Geometry: see drawing. Coordinates: mm, zero at the bounding-box minimum. Coordinates: 2 decimals unless noted, no trailing zeros. Write each loop counter-clockwise with the first axis right and the second up, starting at its lowest first coordinate (ties: lowest second). Pieces come first, ordered by that corner, then holes. Notation, with made-up numbers: (89.25, 1.25) - (126.25, 1.25) arc R14 ccw to (126.25, 27.25) - close; hole circle Ø6 at (21.25, 2). An arc over 180 degrees is marked (long way). Use CSV: the item, a comma, the result in double quotes.
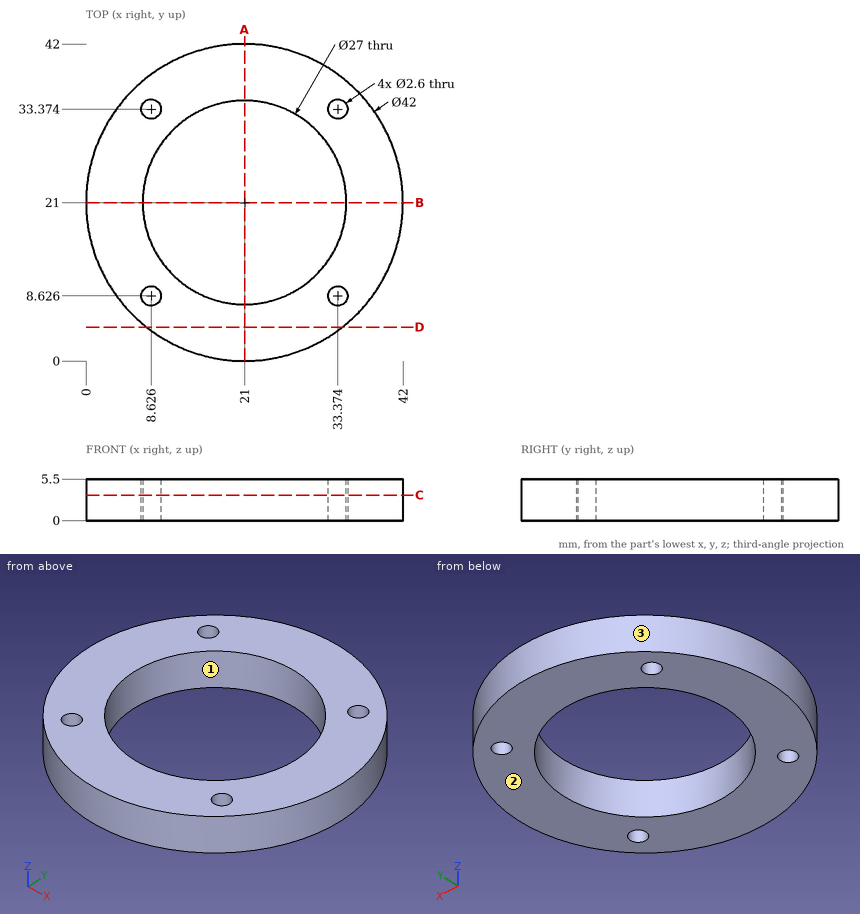
(1) Draft query along Y for the marked faces 1, 2 and 3. Return one class per face: pulls with the +Y half, pulls with the -Y half, needs draft (parallel to the pull), parting line crosses it, or undercut.
Check values:
face 1,"undercut"
face 2,"needs draft"
face 3,"parting line crosses it"
(2) Pin query (flat end, axial travel): pin 1 Ø3 at (x, z) = (32, 2) entering from +Y; pin 2 Ø2 at (x, z) = (24, 1) entering from -Y (1 decimal); pin 3 Ø2 at (x, z) = (9.5, 4.5) entering from +Y. Return the tip coordinate at first contact, or that it passes through.
Check values:
pin 1,"y = 39.73"
pin 2,"y = 0.1"
pin 3,"y = 39.19"
(3) Cut plane C-C on z = 3.35. Return loops of the section in (x, y) (1 decimal).
Check values:
outline,"circle Ø42 at (21, 21); hole circle Ø2.6 at (8.6, 8.6); hole circle Ø2.6 at (8.6, 33.4); hole circle Ø27 at (21, 21); hole circle Ø2.6 at (33.4, 8.6); hole circle Ø2.6 at (33.4, 33.4)"
(4) Cut plane D-D on y = 4.5. Return loops of the section in (x, z), and give its area (3 significant figures).
Check values:
outline,"(8.01, 0) - (33.99, 0) - (33.99, 5.5) - (8.01, 5.5) - close"
area,"143 mm^2"
(5) Cut plane A-A on x = 21. Return loops of the section in (y, z).
Check values:
outline,"(0, 0) - (7.5, 0) - (7.5, 5.5) - (0, 5.5) - close; (34.5, 0) - (42, 0) - (42, 5.5) - (34.5, 5.5) - close"
(6) Ray query, probe 1 along X at (y, z) = (33, 2.3) (1 decimal); probe 2 along Y at (x, z) = (19, 3.7) (1 decimal); probe 3 along X at (y, z) = (22.5, 4.85). Return the intervals inside material, ascending. Write a range as from..to.
Check values:
probe 1,"3.8..7.4, 9.9..14.8, 27.2..32.1, 34.6..38.2"
probe 2,"0.1..7.6, 34.4..41.9"
probe 3,"0.05..7.58, 34.42..41.95"
